Can you work these out from the model? Positions are in its coordinate system, mm. A direction names the side the tool comes from. Give positions to 0.01 mm unless a question says otherwise; leave off trailing zeros. Loops run counter-clockwise (first coordinate to the right, second up) from the corner with the lowest first, then second, coordinate; pieces in that order, holes last. Notation, with made-up numbers: M -11,50 L 35,50 A21 cw 35,58 Z; hole C 45.5,86 d1. An arc over 180 degrees is marked long. Put each result on its own line as item: value. Start each with the question number.
1) For P1, Ø9.5, axis at x = 10.5, y = -12.5, coming from the +Z side (3 decimals); P2, Ø6, axis at y = -35, z = -0.5, coming from the +X side (3 decimals), each with a flat end and sliding along its axis, tell me the tip position at first contact or that it passes through.
2) If we mould it in two halves opening along Y, with no side actions, what happens to faces 1 (the flat face through (9, 131.762, 0)), 2 (the flat face through (15.875, -2, 1)), 3 (the flat face through (10, 42.862, 25))? For each: +Y half, -Y half, draft (parallel to the pull), parting line (faces both ways), or undercut.
3) Imagine slicing it at B-B (y = -80). Write out the boundary of the cut face in (x, z) (3 decimals), then the cut area to 3 significant figures.
4) Imagine slicing it at C-C (z = -6). Write out the boundary of the cut face in (x, y) (1 decimal).
5) Please list where these lines run through material, in increasing order: line 1 along Y through (x, z) = (9, 26); line 2 along Z through (x, y) = (17.25, 57.5) (3 decimals); line 3 along Z through (x, y) = (17, -41) (3 decimals). Write a range as from..to.
6) Imagine slicing it at A-A (x = 9.5). Write out the boundary of the cut face in (y, z) (1 decimal).
7) For faces 4 (the flat face through (9, -88, 28.575)), 5 (the flat face through (10, -1, 22.225)), which set-ups out of +Z, -Z, +X, -X, +Y, -Y let a thin tool reach every point of the face, with its end or its side?
from build123d import *

# Parameters (mm, degrees)
F0_W     = 263.525
F0_H     = 57.15
F1_DEPTH = 19.05
F2_W     = 263.525
F2_H     = 20.701
F3_DEPTH = 3.175
F4_W     = 85.725
F4_H     = 6.35
F5_DEPTH = 19.05


with BuildPart() as f1:
    # F0 (on Right) → F1 (new body)
    with BuildSketch(Plane.YZ):
        Rectangle(F0_W, F0_H)
    extrude(amount=F1_DEPTH)

    # F2 (on face) → F3 (cut)
    with BuildSketch(Plane.YZ.offset(19.05)):
        with Locations((0, 0.8255)):
            Rectangle(F2_W, F2_H)
    extrude(amount=-F3_DEPTH, mode=Mode.SUBTRACT)

    # F4 (on face) → F5 (cut, through all)
    with BuildSketch(Plane.YZ.offset(19.05)):
        with Locations((0, 25.4)):
            Rectangle(F4_W, F4_H)
    extrude(amount=-F5_DEPTH, mode=Mode.SUBTRACT)


solid = f1.part
Recorded:
1. P1: z = 22.225
1. P2: x = 15.875
2. face 1: +Y half
2. face 2: draft
2. face 3: undercut
3. outline: M 0,-28.575 L 19.05,-28.575 L 19.05,-9.525 L 15.875,-9.525 L 15.875,11.176 L 19.05,11.176 L 19.05,28.575 L 0,28.575 Z
3. area: 1,020 mm²
4. outline: M 0,-131.8 L 15.9,-131.8 L 15.9,131.8 L 0,131.8 Z
5. line 1: -131.76..-42.86, 42.86..131.76
5. line 2: -28.575..-9.525, 11.176..28.575
5. line 3: -28.575..-9.525, 11.176..22.225
6. outline: M -131.8,-28.6 L 131.8,-28.6 L 131.8,28.6 L 42.9,28.6 L 42.9,22.2 L -42.9,22.2 L -42.9,28.6 L -131.8,28.6 Z
7. face 4: +Z, +X, -X, +Y, -Y
7. face 5: +Z, +X, -X
